The listing builds one solid part. Answer for the finished solid, in the listing's coordinates (mm). A direction names the side the tool comes from. Give positions to 0.01 mm unless a question says otherwise; leave off trailing zeros. Order: outer loops, then holes, each group sorted by start corner. A loop starts at its lowest first (then second) coordinate and runs counter-clockwise, first axis right, second up. Notation, with made-up numbers: (-30, 59) - (10, 59) arc R23 cw to (10, 97) - close; hole circle Ø5 at (70, 44.5). An arc over 180 degrees is marked (long way). Use a Markdown table: item, result. Add a question column.
1) Find section B-B, the plane y = 0. Determine the outline of the cut face in (x, z), plus the area to 3 significant figures.
2) Find section D-D, the plane z = 1.2. Determine the outline of the cut face in (x, y).
3) Straight lines are drawn through the part: line 1 (Z direction, x = 54, y = 0.8); line 2 (X direction, y = 0.05, z = -0.3); line 3 (X direction, y = 0.05, z = 0.6). For each, find the intervals that lie inside material, in ascending order.
4) Find section A-A, the plane x = 58. Determine the outline of the cut face in (y, z), plus the area to 3 significant figures.
5) The mould has two halves that part along X. Classify faces 1 (the face through (6, 2, -1)), 2 (the face through (56, 0, -2.5)), 3 (the face through (0, 0, 0)): released by +X, released by -X, zero draft, split by the parting line, or undercut.
6) Flat-ended cylindrical pins translate along their axes: pin 1 (1.7 mm diameter, centred on x = 56.5, y = 0.5, fed in from -Z); pin 2 (2 mm diameter, centred on x = 22.5, y = 0.5, fed in from +Z); pin 3 (2 mm diameter, centred on x = 53.5, z = -1.5, fed in from +Y). Find the tip coordinate at first contact, or state that the pin passes through.
7) For faces 4 (the face through (53, 0, 1)), 5 (the face through (59.11, -0.46, -1.23)), 6 (the face through (41, 2, 0)), determine the directions among +Z, -Z, +X, -X, +Y, -Y from which every point of the face is accessible in a straight line to the end or side of a thin tool.
8) Find section C-C, the plane z = -1.05. Determine the outline of the cut face in (x, y), plus the area to 3 significant figures.
from build123d import *

# Parameters (mm, degrees)
F2_W          = 11.2872527242
F2_H          = 5.0563791087
F2_H_2        = 3.2026648214
F3_DEPTH      = 3.001
F3_DEPTH_BACK = 3.001
F4_R          = 1.2
F5_DEPTH      = 3.001


with BuildPart() as f1:
    # F0 (on Front) → F1 (revolve)
    with BuildSketch(Plane.XZ):
        Polygon((0, 3), (0, 0), (61, 0), (61, 3), (51, 3), (51, 2), (32, 2), (32, 3), (26, 3), (26, 2), (6, 2), (6, 3), align=None)
    revolve(axis=Axis((32.858710736, 0, 0), (1, 0, 0)))

    # F2 (on Front) → F3 (cut, two sides)
    with BuildSketch(Plane.XZ) as f3_sk:
        with Locations((58.6436263621, 2.5281895543)):
            Rectangle(F2_W, F2_H)
        with Locations((58.6436263621, -4.1013324107)):
            Rectangle(F2_W, F2_H_2)
    extrude(amount=-F3_DEPTH, mode=Mode.SUBTRACT)
    extrude(f3_sk.sketch, amount=F3_DEPTH_BACK, mode=Mode.SUBTRACT)

    # F4 (on face) → F5 (cut, through all)
    with BuildSketch(Plane.XY):
        with Locations((58, 0)):
            Circle(F4_R)
    extrude(amount=-F5_DEPTH, mode=Mode.SUBTRACT)


solid = f1.part
The answers:
| question | item | result |
|---|---|---|
| 1 | outline | (0, -3) - (6, -3) - (6, -2) - (26, -2) - (26, -3) - (32, -3) - (32, -2) - (51, -2) - (51, -3) - (53, -3) - (53, -2.5) - (56.8, -2.5) - (56.8, 0) - (53, 0) - (53, 3) - (51, 3) - (51, 2) - (32, 2) - (32, 3) - (26, 3) - (26, 2) - (6, 2) - (6, 3) - (0, 3) - close; (59.2, -2.5) - (61, -2.5) - (61, 0) - (59.2, 0) - close |
| 1 | area | 254 mm2 |
| 2 | outline | (0, -2.75) - (6, -2.75) - (6, -1.6) - (26, -1.6) - (26, -2.75) - (32, -2.75) - (32, -1.6) - (51, -1.6) - (51, -2.75) - (53, -2.75) - (53, 2.75) - (51, 2.75) - (51, 1.6) - (32, 1.6) - (32, 2.75) - (26, 2.75) - (26, 1.6) - (6, 1.6) - (6, 2.75) - (0, 2.75) - close |
| 3 | line 1 | -2.5 to 0 |
| 3 | line 2 | 0 to 56.8, 59.2 to 61 |
| 3 | line 3 | 0 to 53 |
| 4 | outline | (-3, 0) arc R3 ccw to (-1.66, -2.5) - (-1.2, -2.5) - (-1.2, 0) - close; (1.2, -2.5) - (1.66, -2.5) arc R3 ccw to (3, 0) - (1.2, 0) - close |
| 4 | area | 7.01 mm2 |
| 5 | face 1 | undercut |
| 5 | face 2 | zero draft |
| 5 | face 3 | released by -X |
| 6 | pin 1 | z = -2.5 |
| 6 | pin 2 | z = 2 |
| 6 | pin 3 | y = 2.96 |
| 7 | face 4 | +Z, +X, +Y, -Y |
| 7 | face 5 | +Z, -Z |
| 7 | face 6 | none |
| 8 | outline | (0, -2.81) - (6, -2.81) - (6, -1.7) - (26, -1.7) - (26, -2.81) - (32, -2.81) - (32, -1.7) - (51, -1.7) - (51, -2.81) - (61, -2.81) - (61, 2.81) - (51, 2.81) - (51, 1.7) - (32, 1.7) - (32, 2.81) - (26, 2.81) - (26, 1.7) - (6, 1.7) - (6, 2.81) - (0, 2.81) - close; hole circle Ø2.4 at (58, 0) |
| 8 | area | 252 mm2 |
